Geometry check sheet. Reference: the model listing, model coordinates, mm. Round coordinates to 2 decimals unless told otherwise and drop trailing zeros. Write each loop counter-clockwise with the first axis right and the second up, starting at its lowest first coordinate (ties: lowest second). Pieces come first, ordered by that corner, then holes. Notation, with made-up numbers: (45, -27.75) - (63, -27.75) arc R5 cw to (63, -20.75) - close; hole circle Ø9 at (85.5, 65.5). An arc over 180 degrees is marked (long way). Return JSON: item names as keys, results as strings.
```python
from build123d import *

# Parameters (mm, degrees)
SKETCH1_W           = 193
SKETCH1_H           = 70
BOSS_EXTRUDE1_DEPTH = 35
SKETCH2_W           = 33
SKETCH2_H           = 70
CUT_EXTRUDE1_DEPTH  = 194
SKETCH3_W           = 35
SKETCH3_H           = 12.5
CUT_EXTRUDE2_DEPTH  = 10


with BuildPart() as part:
    # Sketch1 → Boss-Extrude1 (new body)
    with BuildSketch(Plane(origin=(0, 0, 0), x_dir=(0, 0, -1), z_dir=(1, 0, 0))):
        with Locations((96.5, 35)):
            Rectangle(SKETCH1_W, SKETCH1_H)
    extrude(amount=BOSS_EXTRUDE1_DEPTH)

    # Sketch2 → Cut-Extrude1 (cut, through all)
    with BuildSketch(Plane.XY):
        with Locations((16.5, 35)):
            Rectangle(SKETCH2_W, SKETCH2_H)
    extrude(amount=-CUT_EXTRUDE1_DEPTH, mode=Mode.SUBTRACT)

    # Sketch3 → Cut-Extrude2 (cut)
    with BuildSketch(Plane(origin=(35, 0, 0), x_dir=(0, 0, -1), z_dir=(1, 0, 0))):
        with Locations((175.5, 44.75)):
            Rectangle(SKETCH3_W, SKETCH3_H)
    extrude(amount=-CUT_EXTRUDE2_DEPTH, mode=Mode.SUBTRACT)


solid = part.part
```
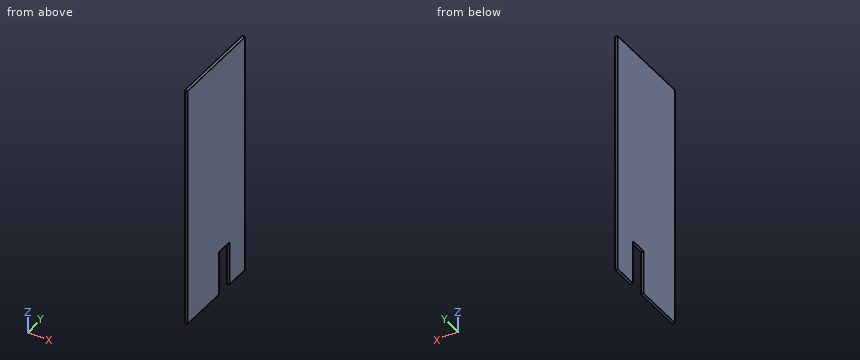
(1) Gauge pin test, flat ends, axial feed: pin 1 (0.6 mm diameter, centred on x = 34, z = -175.5, fed in from -Y); pin 2 (0.6 mm diameter, centred on x = 34, y = 41.5, fed in from -Z). Record the tip position at first contact, or that the pin passes through.
Response values:
{"pin 1": "stops at y = 0", "pin 2": "stops at z = -158"}
(2) Section check A-A, the plane x = 34.45. Enter the section's corners in (y, z), plus the area to 3 significant figures.
Response values:
{"outline": "(0, -193) - (38.5, -193) - (38.5, -158) - (51, -158) - (51, -193) - (70, -193) - (70, 0) - (0, 0) - close", "area": "13,100 mm^2"}
(3) Material ranges on line 1 along Y through (x, z) = (33.8, -161.5), recorded low to high. Write a range as [from, to].
Response values:
{"line 1": "y = [0, 38.5], [51, 70]"}
